```python
from build123d import *

# Parameters (mm, degrees)
CHAMFER1_SIZE      = 2
SKETCH2_RX         = 8.815168497
SKETCH2_RY         = 6.763008786
SKETCH2_RX_2       = 5.446652698
SKETCH2_RY_2       = 3.762863515
CUT_EXTRUDE1_DEPTH = 4
CIRPATTERN1_COUNT  = 3
SKETCH3_R          = 12.054961978
CUT_EXTRUDE2_DEPTH = 20
CUT_EXTRUDE3_DEPTH = 46.890031658
CIRPATTERN3_COUNT  = 2
CIRPATTERN3_ANGLE  = 90
SKETCH5_R          = 1.75
CUT_EXTRUDE4_DEPTH = 1


with BuildPart() as part:
    # Sketch1 → Revolve1 (revolve)
    with BuildSketch(Plane.XY):
        Polygon((-3.2, 0), (-13.85, 0), (-13.85, 7.1), (-12.85, 7.1), (-12.85, 7.6), (-13.85, 7.6), (-13.85, 32), (-4, 32), (-4, 36), (-3, 36), (-3, 41.5), (0, 41.5), (0, -2.5), (-3.2, -2.5), align=None)
    revolve(axis=Axis((0, 41.5, 0), (0, -1, 0)))

    # Chamfer1
    chamfer1_edges = [part.edges().sort_by_distance(p)[0] for p in [
        (13.85, 0, 0),
        (13.85, 32, 0),
    ]]
    chamfer(chamfer1_edges, length=CHAMFER1_SIZE)

    # Sketch2 → Cut-Extrude1 (cut)
    with BuildSketch(Plane(origin=(0, 32, 0), x_dir=(1, 0, 0), z_dir=(0, 1, 0))):
        with Locations(Location((0, -13.85), (0, 0, 90))):
            Ellipse(SKETCH2_RX, SKETCH2_RY)
        with Locations(Location((0, 13.85), (0, 0, -90))):
            Ellipse(SKETCH2_RX_2, SKETCH2_RY_2)
        with Locations(Location((-77.957366116, 6.373706544), (0, 0, 90))):
            Ellipse(SKETCH2_RX, SKETCH2_RY)
        with Locations(Location((-77.957366116, 34.073706544), (0, 0, 90))):
            Ellipse(SKETCH2_RX_2, SKETCH2_RY_2)
    cut_extrude1 = extrude(amount=-CUT_EXTRUDE1_DEPTH, mode=Mode.SUBTRACT)

    # CirPattern1: Cut-Extrude1 ×3 about axis
    cirpattern1_axis = Axis((0, 41.5, 0), (0, 1, 0))
    for i in range(1, CIRPATTERN1_COUNT):
        add(cut_extrude1.rotate(cirpattern1_axis, i * 360 / CIRPATTERN1_COUNT), mode=Mode.SUBTRACT)

    # Sketch3 → Cut-Extrude2 (cut)
    with BuildSketch(Plane(origin=(0, 28, 0), x_dir=(1, 0, 0), z_dir=(0, 1, 0))):
        with Locations(Location((0, 0, 0), (0, 0, 180))):
            Circle(SKETCH3_R)
    extrude(amount=-CUT_EXTRUDE2_DEPTH, mode=Mode.SUBTRACT)

    # Sketch4 → Cut-Extrude3 (cut, symmetric)
    with BuildSketch(Plane(origin=(0, 0, 0), x_dir=(0, 0, -1), z_dir=(1, 0, 0))):
        with BuildLine():
            Line((-6.75, 6), (6.75, 6))
            ThreePointArc((6.75, 6), (8.25, 4.5), (6.75, 3))
            Line((6.75, 3), (-6.75, 3))
            ThreePointArc((-6.75, 3), (-8.25, 4.5), (-6.75, 6))
        make_face()
    cut_extrude3 = extrude(amount=CUT_EXTRUDE3_DEPTH, both=True, mode=Mode.SUBTRACT)

    # CirPattern3: Cut-Extrude3 ×2 about axis
    cirpattern3_axis = Axis((0, 41.5, 0), (0, 1, 0))
    for i in range(1, CIRPATTERN3_COUNT):
        add(cut_extrude3.rotate(cirpattern3_axis, i * CIRPATTERN3_ANGLE / (CIRPATTERN3_COUNT - 1)), mode=Mode.SUBTRACT)

    # Sketch5 → Cut-Extrude4 (cut)
    with BuildSketch(Plane.XZ):
        with Locations((-9.5, 0)):
            Circle(SKETCH5_R)
        with Locations((0, 8)):
            Circle(SKETCH5_R)
        with Locations((9.5, 0)):
            Circle(SKETCH5_R)
        with Locations((0, -8)):
            Circle(SKETCH5_R)
    extrude(amount=-CUT_EXTRUDE4_DEPTH, mode=Mode.SUBTRACT)


solid = part.part
```
Verification items for the finished model (mm, model axes). A direction names the side the tool comes from. Coordinates: 2 decimals unless noted, no trailing zeros. Loops run counter-clockwise (first coordinate to the right, second up) from the corner with the lowest first, then second, coordinate; pieces in that order, holes last. Notation, with made-up numbers: (76.25, 60) -> (90.25, 60) arc R13 ccw to (90.25, 70) -> close; hole circle Ø2 at (38.5, -13.5). An arc over 180 degrees is marked (long way). Put each result on its own line as item: value.
1. Section check A-A, the plane y = 11. Record the boundary of the cut face in (x, z).
Result set:
outline: circle Ø27.7 at (0, 0); hole circle Ø24.11 at (0, 0)
2. Section check B-B, the plane x = 0.5. Give the number of separate pieces and of enclosed holes in the cut face, then the cut area to 3 significant figures.
Result set:
separate pieces: 3
enclosed holes: 0
area: 333 mm^2
3. Gauge pin test, flat ends, axial feed: P1, Ø10, axis at x = 5, z = 10.5, coming from the -Y side; P2, Ø4.5, axis at x = 0, z = -8, coming from the +Y side; P3, Ø1.5, axis at y = 32.5, z = 9.5, coming from the -X side; P4, Ø1, axis at y = 4.5, z = -6.5, coming from the +X side. Record the tip position at first contact, or that the pin passes through.
Result set:
P1: stops at y = 0
P2: stops at y = 32
P3: stops at x = -7.8
P4: passes through
4. Tool access check on faces 1 (the face through (10.197, 7.354, 7.819)), 2 (the face through (0.867, 34.028, 3.905)), 3 (the face through (9, 1, 0)), 4 (the face through (8.25, 4.47, 9.38)). Record the directions out of +Z, -Z, +X, -X, +Y, -Y that give a thin tool (end or side, any length) a straight path to the whole face; none if there is none.
Result set:
face 1: none
face 2: +Y
face 3: -Y
face 4: +Z, -Z
5. Mould release check, pull along X, two halves, no side actions. Record for faces 5 (the face through (0, 28, 13)), 6 (the face through (9.46, 4.53, -8.25)), 7 (the face through (11.169, 0.493, 0.526)), 8 (the face through (-7.61, 31.01, 10.34)): pulls with the +X half, pulls with the -X half, needs draft (parallel to the pull), parting line crosses it, or undercut.
Result set:
face 5: undercut
face 6: needs draft
face 7: undercut
face 8: pulls with the -X half
6. Thickness scan on line 1 (Y direction, x = -0.25, z = -1.75); line 2 (Y direction, x = -4.25, z = 0.5); line 3 (Y direction, x = -10.75, z = 4.5). Record the ranges inside material, lowest first.
Result set:
line 1: y = -2.5 to 3, 6 to 8, 28 to 41.5
line 2: y = 0 to 3, 6 to 8, 28 to 32
line 3: y = 0 to 3, 6 to 8
7. Section check C-C, the plane y = 34.5. Record the boundary of the cut face in (x, z), then the cut area to 3 significant figures.
Result set:
outline: circle Ø8 at (0, 0)
area: 50.3 mm^2
